The figure shows three views and two pictorial views of one solid part (mm, origin at its lowest corner). Answer the questions. A direction names the side the tool comes from. Coordinates: 2 decimals unless noted, no trailing zeros. Write each loop counter-clockwise with the first axis right and the second up, starting at its lowest first coordinate (ties: lowest second). Pieces come first, ordered by that corner, then holes. Notation, with made-up numbers: M 55,10 L 89,10 A22 cw 89,23 Z; hole C 42,-34.75 d1. An arc over 180 degrees is marked long. Use CSV: the item, a comma, the result in double quotes.
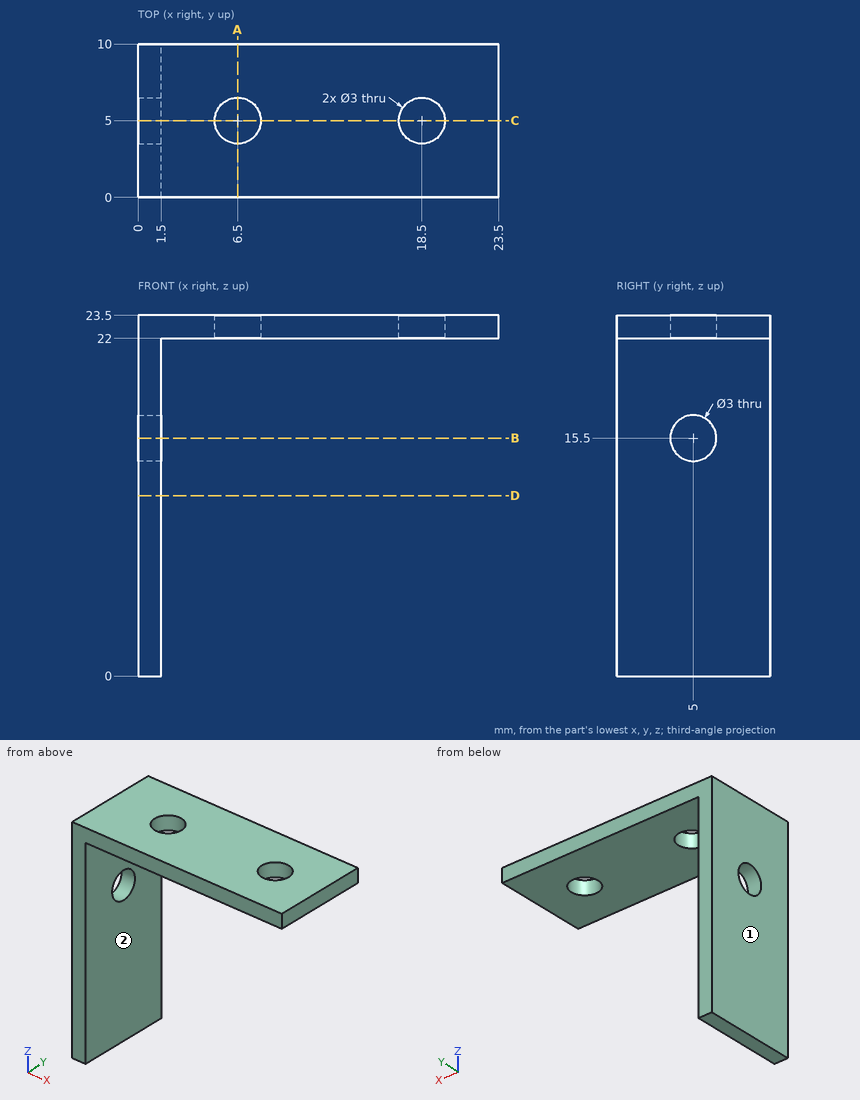
Item 1: The part is cut by section A-A (x = 6.5). Write down the section's boundary in (y, z), then the cut area to 3 significant figures.
Answer:
outline,"M 0,22 L 3.5,22 L 3.5,23.5 L 0,23.5 Z; M 6.5,22 L 10,22 L 10,23.5 L 6.5,23.5 Z"
area,"10.5 mm2"
Item 2: Given pin 1 (3.5 mm diameter, centred on y = 5, z = 15.5, fed in from +X); pin 2 (5 mm diameter, centred on x = 12.5, y = 7.5, fed in from -Z); pin 3 (2.5 mm diameter, centred on x = 6.5, y = 5, fed in from +Z), each flat-ended and moving along its own axis, determine where each tip first touches the part or whether it passes through.
Answer:
pin 1,"stops at x = 1.5"
pin 2,"stops at z = 22"
pin 3,"passes through"
Item 3: The part is cut by section C-C (y = 5). Write down the section's boundary in (x, z).
Answer:
outline,"M 0,0 L 1.5,0 L 1.5,14 L 0,14 Z; M 0,17 L 1.5,17 L 1.5,22 L 5,22 L 5,23.5 L 0,23.5 Z; M 8,22 L 17,22 L 17,23.5 L 8,23.5 Z; M 20,22 L 23.5,22 L 23.5,23.5 L 20,23.5 Z"
Item 4: The part is cut by section B-B (z = 15.5). Write down the section's boundary in (x, y), then the cut area to 3 significant figures.
Answer:
outline,"M 0,0 L 1.5,0 L 1.5,3.5 L 0,3.5 Z; M 0,6.5 L 1.5,6.5 L 1.5,10 L 0,10 Z"
area,"10.5 mm2"
Item 5: The part is cut by section D-D (z = 11.75). Write down the section's boundary in (x, y).
Answer:
outline,"M 0,0 L 1.5,0 L 1.5,10 L 0,10 Z"
Item 6: A tool of negligible diameter and unlimited length cuts with its end or side. For the marked faces 1 and 2, from which of +Z, -Z, +X, -X, +Y, -Y can it reach the whole face along a straight path? Write none if from no direction.
Answer:
face 1,"+Z, -Z, -X, +Y, -Y"
face 2,"-Z, +X, +Y, -Y"
Item 7: Consider probe 1 along Y at (x, z) = (0.35, 15.5); probe 2 along Z at (x, y) = (16.5, 8.75); probe 3 along X at (y, z) = (4.5, 17.5). Determine where each line is inside the solid, lowest interval first.
Answer:
probe 1,"y = 0 to 3.5, 6.5 to 10"
probe 2,"z = 22 to 23.5"
probe 3,"x = 0 to 1.5"
